Geometry check sheet. Reference: the model listing, model coordinates, mm. A direction names the side the tool comes from. Round coordinates to 2 decimals unless told otherwise and drop trailing zeros. Loops run counter-clockwise (first coordinate to the right, second up) from the corner with the lowest first, then second, coordinate; pieces in that order, holes last. Notation, with made-up numbers: (-13.75, 39.5) -> (-3.75, 39.5) arc R25 cw to (-3.75, 63.5) -> close; hole circle Ø3 at (-28, 83). An arc over 180 degrees is marked (long way). Use one line per item in the form item = value.
from build123d import *

# Parameters (mm, degrees)
SKETCH_2_W          = 60.94
SKETCH_2_H          = 20
EXTRUDE_1_DEPTH     = 1
SKETCH_3_W          = 1
SKETCH_3_H          = 20
EXTRUDE_2_DEPTH     = 32.81
SKETCH_4_W          = 1
SKETCH_4_H          = 20
EXTRUDE_3_DEPTH     = 32.81
SKETCH_9_W          = 20
SKETCH_9_H          = 1
EXTRUDE_8_DEPTH     = 9.12
SKETCH_10_W         = 20
SKETCH_10_H         = 1
EXTRUDE_9_DEPTH     = 9.12
SKETCH_13_R         = 1.6
CUT_EXTRUDE_2_DEPTH = 1
SKETCH_14_R         = 1.6
CUT_EXTRUDE_3_DEPTH = 1
SKETCH_15_R         = 1.6
CUT_EXTRUDE_4_DEPTH = 1
SKETCH_16_R         = 1.6
CUT_EXTRUDE_5_DEPTH = 1
SKETCH_17_R         = 1.6
CUT_EXTRUDE_6_DEPTH = 1


with BuildPart() as part:
    # ｽｹｯﾁ2 → ﾎﾞｽ - 押し出し1 (new body)
    with BuildSketch(Plane(origin=(0, 0, 0), x_dir=(1, 0, 0), z_dir=(0, 1, 0))):
        with Locations((30.47, 10)):
            Rectangle(SKETCH_2_W, SKETCH_2_H)
    extrude(amount=EXTRUDE_1_DEPTH)

    # ｽｹｯﾁ3 → ﾎﾞｽ - 押し出し2 (add)
    with BuildSketch(Plane(origin=(0, 1, 0), x_dir=(1, 0, 0), z_dir=(0, 1, 0))):
        with Locations((60.44, 10)):
            Rectangle(SKETCH_3_W, SKETCH_3_H)
    extrude(amount=EXTRUDE_2_DEPTH)

    # ｽｹｯﾁ4 → ﾎﾞｽ - 押し出し3 (add)
    with BuildSketch(Plane(origin=(0, 1, 0), x_dir=(1, 0, 0), z_dir=(0, 1, 0))):
        with Locations((0.5, 10)):
            Rectangle(SKETCH_4_W, SKETCH_4_H)
    extrude(amount=EXTRUDE_3_DEPTH)

    # ｽｹｯﾁ9 → ﾎﾞｽ - 押し出し8 (add)
    with BuildSketch(Plane.ZY.offset(-59.94)):
        with Locations((-10, 33.31)):
            Rectangle(SKETCH_9_W, SKETCH_9_H)
    extrude(amount=EXTRUDE_8_DEPTH)

    # ｽｹｯﾁ10 → ﾎﾞｽ - 押し出し9 (add)
    with BuildSketch(Plane(origin=(1, 0, 0), x_dir=(0, 0, -1), z_dir=(1, 0, 0))):
        with Locations((10, 33.31)):
            Rectangle(SKETCH_10_W, SKETCH_10_H)
    extrude(amount=EXTRUDE_9_DEPTH)

    # ｽｹｯﾁ13 → ｶｯﾄ - 押し出し2 (cut)
    with BuildSketch(Plane(origin=(0, 33.81, 0), x_dir=(1, 0, 0), z_dir=(0, 1, 0))):
        with Locations((55.49, 5.12)):
            Circle(SKETCH_13_R)
    extrude(amount=-CUT_EXTRUDE_2_DEPTH, mode=Mode.SUBTRACT)

    # ｽｹｯﾁ14 → ｶｯﾄ - 押し出し3 (cut)
    with BuildSketch(Plane(origin=(0, 33.81, 0), x_dir=(1, 0, 0), z_dir=(0, 1, 0))):
        with Locations((55.49, 14.88)):
            Circle(SKETCH_14_R)
    extrude(amount=-CUT_EXTRUDE_3_DEPTH, mode=Mode.SUBTRACT)

    # ｽｹｯﾁ15 → ｶｯﾄ - 押し出し4 (cut)
    with BuildSketch(Plane(origin=(0, 33.81, 0), x_dir=(1, 0, 0), z_dir=(0, 1, 0))):
        with Locations((5.45, 5.12)):
            Circle(SKETCH_15_R)
    extrude(amount=-CUT_EXTRUDE_4_DEPTH, mode=Mode.SUBTRACT)

    # ｽｹｯﾁ16 → ｶｯﾄ - 押し出し5 (cut)
    with BuildSketch(Plane(origin=(0, 33.81, 0), x_dir=(1, 0, 0), z_dir=(0, 1, 0))):
        with Locations((5.45, 14.88)):
            Circle(SKETCH_16_R)
    extrude(amount=-CUT_EXTRUDE_5_DEPTH, mode=Mode.SUBTRACT)

    # ｽｹｯﾁ17 → ｶｯﾄ - 押し出し6 (cut)
    with BuildSketch(Plane(origin=(0, 0, 0), x_dir=(-1, 0, 0), z_dir=(0, -1, 0))):
        with Locations((-41.55, 10)):
            Circle(SKETCH_17_R)
    extrude(amount=-CUT_EXTRUDE_6_DEPTH, mode=Mode.SUBTRACT)


solid = part.part
1. Section check A-A (x = 5.45). Record the boundary of the cut face in (y, z).
Return value:
outline = (0, -20) -> (1, -20) -> (1, 0) -> (0, 0) -> close; (32.81, -20) -> (33.81, -20) -> (33.81, -16.48) -> (32.81, -16.48) -> close; (32.81, -13.28) -> (33.81, -13.28) -> (33.81, -6.72) -> (32.81, -6.72) -> close; (32.81, -3.52) -> (33.81, -3.52) -> (33.81, 0) -> (32.81, 0) -> close
2. Section check D-D (x = 41.55). Record the boundary of the cut face in (y, z).
Return value:
outline = (0, -20) -> (1, -20) -> (1, -11.6) -> (0, -11.6) -> close; (0, -8.4) -> (1, -8.4) -> (1, 0) -> (0, 0) -> close
3. Tool access check on faces 4 (the cylindrical face through (43.15, 0.49, -10.07)), 5 (the flat face through (59.94, 17, -10)), 6 (the cylindrical face through (54.22, 33.32, -4.15)). Record the directions out of +Z, -Z, +X, -X, +Y, -Y that give a thin tool (end or side, any length) a straight path to the whole face; none if there is none.
Return value:
face_4 = +Y, -Y
face_5 = +Z, -Z
face_6 = +Y
4. Section check B-B (z = -10). Record the boundary of the cut face in (x, y).
Return value:
outline = (0, 0) -> (39.95, 0) -> (39.95, 1) -> (1, 1) -> (1, 32.81) -> (10.12, 32.81) -> (10.12, 33.81) -> (0, 33.81) -> close; (43.15, 0) -> (60.94, 0) -> (60.94, 33.81) -> (50.82, 33.81) -> (50.82, 32.81) -> (59.94, 32.81) -> (59.94, 1) -> (43.15, 1) -> close
5. Gauge pin test, flat end, axial feed: pin 1 (2.5 mm diameter, centred on x = 5.45, z = -14.88, fed in from +Y). Record the tip position at first contact, or that the pin passes through.
Return value:
pin_1 = 1
6. Section check C-C (y = 31.5). Record the boundary of the cut face in (x, z), then the cut area to 3 significant figures.
Return value:
outline = (0, -20) -> (1, -20) -> (1, 0) -> (0, 0) -> close; (59.94, -20) -> (60.94, -20) -> (60.94, 0) -> (59.94, 0) -> close
area = 40.0 mm2
7. Mould release check, pull along Z, two halves, no side actions. Record for faces 1 (the flat face through (56, 33.81, -10)), 2 (the flat face through (19, 0.5, -20)), 3 (the cylindrical face through (6.31, 33.32, -16.23)): released by +Z, released by -Z, zero draft, split by the parting line, or undercut.
Return value:
face_1 = zero draft
face_2 = released by -Z
face_3 = undercut
8. Material ranges on line 1 along Z through (x, y) = (55.49, 33.45); line 2 along X through (y, z) = (33.55, -14.88); line 3 along X through (y, z) = (27.5, -1.75), recorded low to high.
Return value:
line_1 = -20 to -16.48, -13.28 to -6.72, -3.52 to 0
line_2 = 0 to 3.85, 7.05 to 10.12, 50.82 to 53.89, 57.09 to 60.94
line_3 = 0 to 1, 59.94 to 60.94
